Part model, mm, in its own coordinate system. Round coordinates to 2 decimals unless told otherwise and drop trailing zeros. Write each loop counter-clockwise with the first axis right and the second up, starting at its lowest first coordinate (ties: lowest second). Pieces come first, ordered by that corner, then holes. Notation, with made-up numbers: M -4,74.5 L 20,74.5 A37 cw 20,110.5 Z; hole C 8.25,-14.75 d3. An arc over 180 degrees is marked long. Answer as a JSON object with one key per item and string values. Group by question number.
1. Band-saw the part on B-B, the plane z = 0.7. Write the cut outline in (x, y).
2. Band-saw the part on D-D, the plane y = -7.5. Write the cut outline in (x, z).
3. Drop a flat-ended pin along its axis: pin 1 (2.5 mm diameter, centred on x = -5.72, y = -3.89, fed in from -Z). Give the stop position or say it passes through.
4. Band-saw the part on A-A, the plane y = -4.75. Write the cut outline in (x, z), plus the area to 3 significant figures.
5. Two-plate mould, pull along X, no slides. Class faces 1 (the face through (0.31, -14.88, 0.49)), 2 (the face through (-6.822, -2.878, 0.493)), 3 (the face through (3, -4, 1)), 4 (the face through (0.35, -5.844, 0.493)): +X half, -X half, draft (parallel to the pull), parting line (faces both ways), or undercut.
6. Band-saw the part on C-C, the plane x = -2.75. Write the cut outline in (y, z), plus the area to 3 significant figures.
7. Drill centre lines: line 1 (X direction, y = -4, z = 0.15); line 2 (X direction, y = -5.25, z = 0.5); line 3 (Y direction, x = 1.5, z = 0.1). Where is each one in solid material? Low to high. Write a range as from..to.
from build123d import *

# Parameters (mm, degrees)
SKETCH_1_R          = 11
SKETCH_1_R_2        = 1.5
SKETCH_1_R_3        = 2
EXTRUDE_1_DEPTH     = 1
SKETCH_2_R          = 1
CUT_EXTRUDE_1_DEPTH = 10


with BuildPart() as part:
    # 草图1 → 凸台-拉伸1 (new body)
    with BuildSketch(Plane.XY):
        with Locations((0.783567134, -3.891783567)):
            Circle(SKETCH_1_R)
        with Locations((-5.716432866, -3.891783567)):
            Circle(SKETCH_1_R_2, mode=Mode.SUBTRACT)
        with Locations(Location((7.283567134, -3.891783567, 0), (0, 0, 180))):
            Circle(SKETCH_1_R_2, mode=Mode.SUBTRACT)
        with Locations((0.783567134, -3.891783567)):
            Circle(SKETCH_1_R_3, mode=Mode.SUBTRACT)
    extrude(amount=EXTRUDE_1_DEPTH)

    # 草图2 → 切除-拉伸1 (cut)
    with BuildSketch(Plane.XY.offset(1)):
        with Locations((0.783567134, 7.108216433)):
            Circle(SKETCH_2_R)
    extrude(amount=-CUT_EXTRUDE_1_DEPTH, mode=Mode.SUBTRACT)


solid = part.part
Worked answers:
{
 "1": {"outline": "M -0.22,7.06 A11 ccw long 1.78,7.06 A1 cw Z; hole C -5.72,-3.89 d3; hole C 0.78,-3.89 d4; hole C 7.28,-3.89 d3"},
 "2": {"outline": "M -9.61,0 L 11.17,0 L 11.17,1 L -9.61,1 Z"},
 "3": {"pin 1": "passes through"},
 "4": {"outline": "M -10.18,0 L -6.95,0 L -6.95,1 L -10.18,1 Z; M -4.49,0 L -1.02,0 L -1.02,1 L -4.49,1 Z; M 2.59,0 L 6.05,0 L 6.05,1 L 2.59,1 Z; M 8.51,0 L 11.75,0 L 11.75,1 L 8.51,1 Z", "area": "13.4 mm^2"},
 "5": {"face 1": "parting line", "face 2": "undercut", "face 3": "draft", "face 4": "undercut"},
 "6": {"outline": "M -14.31,0 L 6.53,0 L 6.53,1 L -14.31,1 Z", "area": "20.8 mm^2"},
 "7": {"line 1": "x = -10.22..-7.21, -4.22..-1.21, 2.78..5.79, 8.78..11.78", "line 2": "x = -10.13..-6.35, -5.08..-0.68, 2.25..6.65, 7.92..11.7", "line 3": "y = -14.87..-5.76, -2.02..6.41"}
}
